Input: part model. Units: mm. Frame: model coordinates. A direction names the side the tool comes from. Give positions to 0.01 mm unless a question says otherwise; leave off trailing zeros. Write each loop counter-clockwise with the first axis right and the second up, starting at its lowest first coordinate (ties: lowest second). Pieces come first, ordered by that corner, then holes. Notation, with made-up numbers: (65, 50.5) -> (78, 50.5) arc R38 cw to (78, 89.5) -> close; hole circle Ø9 at (-1.75, 51.5). An arc over 180 degrees is marked (long way). Return JSON: item names as keys, results as strings. Group by question number.
Item 1: Section D-D, the plane y = -28.5. Return loops of the section in (x, z), then the cut area to 3 significant figures.
Item 2: Pin query (flat end, axial travel): P1, Ø4, axis at y = -44.5, z = 65.5, coming from the +X side; P2, Ø3, axis at y = -19.12, z = 75.53, coming from the +X side; P3, Ø2, axis at y = -19.12, z = 6, coming from the -X side. Return the tip coordinate at first contact, or that it passes through.
Item 3: Set-up query: faces 4 (the face through (1.85, -58.32, 1.63)), 5 (the face through (0.37, 0.61, -0.47)). Return all of +Z, -Z, +X, -X, +Y, -Y with unobstructed straight access to the full face (end or side cutting, diameter ignored); none if empty.
Item 4: Line query: line 1 (Z direction, x = 0.7, y = -19.12); line 2 (Y direction, x = -2, z = 6); line 3 (Z direction, x = -1.5, y = -19.12). Output: solid intervals per line, ascending. Write a range as [from, to].
Item 5: Mould query, pull axis Z, two halves, no side actions, for faces 1 (the face through (1.85, -58.22, 80)), 2 (the face through (-3, -29, 41)), 3 (the face through (0, -30, -3.25)). Classes: released by +Z, released by -Z, zero draft, split by the parting line, or undercut.
Item 6: Section A-A, the plane y = -19.12. Return loops of the section in (x, z).
Item 7: Section B-B, the plane x = -1. Return loops of the section in (y, z).
Item 8: Section C-C, the plane z = 54. Return loops of the section in (x, y), then the cut area to 3 significant figures.
from build123d import *

# Parameters (mm, degrees)
BOSS_EXTRUDE1_DEPTH = 3
SKETCH1_3_R         = 4.25
SKETCH1_3_R_2       = 1.25
BOSS_EXTRUDE2_DEPTH = 2
BOSS_EXTRUDE3_START = 3.64
BOSS_EXTRUDE3_DEPTH = 3.64
CUT_EXTRUDE1_REACH  = 107.747
SKETCH1_5_R         = 1.25


with BuildPart() as part:
    # Sketch1 → Boss-Extrude1 (new body)
    with BuildSketch(Plane(origin=(0, 0, 0), x_dir=(0, 0, -1), z_dir=(1, 0, 0))):
        with BuildLine():
            Line((-6, 3.25), (-75.53, 3.25))
            ThreePointArc((-75.53, 3.25), (-82.070737726, 0.540737726), (-84.78, -6))
            Line((-84.78, -6), (-84.78, -53.85))
            ThreePointArc((-84.78, -53.85), (-82.070737726, -60.390737726), (-75.53, -63.1))
            Line((-75.53, -63.1), (-6, -63.1))
            ThreePointArc((-6, -63.1), (0.540737726, -60.390737726), (3.25, -53.85))
            Line((3.25, -53.85), (3.25, -6))
            ThreePointArc((3.25, -6), (0.540737726, 0.540737726), (-6, 3.25))
        make_face()
    extrude(amount=-BOSS_EXTRUDE1_DEPTH)

    # Sketch1_3 → Boss-Extrude2 (add)
    # profile 1 of 4: a face of its own
    with BuildSketch(Plane(origin=(0, 0, 0), x_dir=(0, 0, -1), z_dir=(1, 0, 0))):
        with Locations(Location((-75.53, -19.12, 0), (0, 0, 180))):
            Circle(SKETCH1_3_R)
        with Locations((-75.53, -19.12)):
            Circle(SKETCH1_3_R_2, mode=Mode.SUBTRACT)
    # profile 2 of 4: a face of its own
    with BuildSketch(Plane(origin=(0, 0, 0), x_dir=(0, 0, -1), z_dir=(1, 0, 0))):
        with Locations(Location((-6, -19.12, 0), (0, 0, 180))):
            Circle(SKETCH1_3_R)
        with Locations((-6, -19.12)):
            Circle(SKETCH1_3_R_2, mode=Mode.SUBTRACT)
    # profile 3 of 4: a face of its own
    with BuildSketch(Plane(origin=(0, 0, 0), x_dir=(0, 0, -1), z_dir=(1, 0, 0))):
        with Locations(Location((-6, -42.05, 0), (0, 0, 180))):
            Circle(SKETCH1_3_R)
        with Locations((-6, -42.05)):
            Circle(SKETCH1_3_R_2, mode=Mode.SUBTRACT)
    # profile 4 of 4: a face of its own
    with BuildSketch(Plane(origin=(0, 0, 0), x_dir=(0, 0, -1), z_dir=(1, 0, 0))):
        with Locations(Location((-75.53, -42.05, 0), (0, 0, 180))):
            Circle(SKETCH1_3_R)
        with Locations((-75.53, -42.05)):
            Circle(SKETCH1_3_R_2, mode=Mode.SUBTRACT)
    extrude(amount=BOSS_EXTRUDE2_DEPTH)

    # Sketch1_4 → Boss-Extrude3 (add)
    with BuildSketch(Plane(origin=(0, 0, 0), x_dir=(0, 0, -1), z_dir=(1, 0, 0)).offset(BOSS_EXTRUDE3_START)):
        with BuildLine():
            ThreePointArc((-6, 3.25), (0.540737726, 0.540737726), (3.25, -6))
            Line((3.25, -6), (3.25, -53.85))
            ThreePointArc((3.25, -53.85), (0.540737726, -60.390737726), (-6, -63.1))
            Line((-6, -63.1), (-75.53, -63.1))
            ThreePointArc((-75.53, -63.1), (-82.070737726, -60.390737726), (-84.78, -53.85))
            Line((-84.78, -53.85), (-84.78, -6))
            ThreePointArc((-84.78, -6), (-82.070737726, 0.540737726), (-75.53, 3.25))
            Line((-75.53, 3.25), (-6, 3.25))
        make_face()
        with BuildLine():
            Line((-6, 0.25), (-75.53, 0.25))
            ThreePointArc((-75.53, 0.25), (-79.949417382, -1.580582618), (-81.78, -6))
            Line((-81.78, -6), (-81.78, -53.85))
            ThreePointArc((-81.78, -53.85), (-79.949417382, -58.269417382), (-75.53, -60.1))
            Line((-75.53, -60.1), (-6, -60.1))
            ThreePointArc((-6, -60.1), (-1.580582618, -58.269417382), (0.25, -53.85))
            Line((0.25, -53.85), (0.25, -6))
            ThreePointArc((0.25, -6), (-1.580582618, -1.580582618), (-6, 0.25))
        make_face(mode=Mode.SUBTRACT)
    extrude(amount=-BOSS_EXTRUDE3_DEPTH)

    # Sketch1_5 → Cut-Extrude1 (cut, up to next)
    with BuildSketch(Plane(origin=(0, 0, 0), x_dir=(0, 0, -1), z_dir=(1, 0, 0)), mode=Mode.PRIVATE) as cut_extrude1_sk1:
        with Locations(Location((-6, -19.12, 0), (0, 0, 180))):
            Circle(SKETCH1_5_R)
    cut_extrude1_tool1 = extrude(cut_extrude1_sk1.sketch, amount=-CUT_EXTRUDE1_REACH, mode=Mode.PRIVATE) & part.part
    # Sketch1_5 → Cut-Extrude1 (cut, up to next)
    with BuildSketch(Plane(origin=(0, 0, 0), x_dir=(0, 0, -1), z_dir=(1, 0, 0)), mode=Mode.PRIVATE) as cut_extrude1_sk2:
        with Locations(Location((-6, -42.05, 0), (0, 0, 180))):
            Circle(SKETCH1_5_R)
    cut_extrude1_tool2 = extrude(cut_extrude1_sk2.sketch, amount=-CUT_EXTRUDE1_REACH, mode=Mode.PRIVATE) & part.part
    # Sketch1_5 → Cut-Extrude1 (cut, up to next)
    with BuildSketch(Plane(origin=(0, 0, 0), x_dir=(0, 0, -1), z_dir=(1, 0, 0)), mode=Mode.PRIVATE) as cut_extrude1_sk3:
        with Locations(Location((-75.53, -19.12, 0), (0, 0, 180))):
            Circle(SKETCH1_5_R)
    cut_extrude1_tool3 = extrude(cut_extrude1_sk3.sketch, amount=-CUT_EXTRUDE1_REACH, mode=Mode.PRIVATE) & part.part
    # Sketch1_5 → Cut-Extrude1 (cut, up to next)
    with BuildSketch(Plane(origin=(0, 0, 0), x_dir=(0, 0, -1), z_dir=(1, 0, 0)), mode=Mode.PRIVATE) as cut_extrude1_sk4:
        with Locations(Location((-75.53, -42.05, 0), (0, 0, 180))):
            Circle(SKETCH1_5_R)
    cut_extrude1_tool4 = extrude(cut_extrude1_sk4.sketch, amount=-CUT_EXTRUDE1_REACH, mode=Mode.PRIVATE) & part.part
    add(cut_extrude1_tool1.solids().sort_by_distance((0, -19.12, 6))[0], mode=Mode.SUBTRACT)
    add(cut_extrude1_tool2.solids().sort_by_distance((0, -42.05, 6))[0], mode=Mode.SUBTRACT)
    add(cut_extrude1_tool3.solids().sort_by_distance((0, -19.12, 75.53))[0], mode=Mode.SUBTRACT)
    add(cut_extrude1_tool4.solids().sort_by_distance((0, -42.05, 75.53))[0], mode=Mode.SUBTRACT)


solid = part.part
Answer below:
{
 "1": {"outline": "(-3, -3.25) -> (3.64, -3.25) -> (3.64, -0.25) -> (0, -0.25) -> (0, 81.78) -> (3.64, 81.78) -> (3.64, 84.78) -> (-3, 84.78) -> close", "area": "286 mm2"},
 "2": {"P1": "stops at x = 0", "P2": "stops at x = 2", "P3": "passes through"},
 "3": {"face 4": "+X", "face 5": "-Z, +X, -X, +Y"},
 "4": {"line 1": "z = [-3.25, -0.25], [1.75, 4.75], [7.25, 10.25], [71.28, 74.28], [76.78, 79.78], [81.78, 84.78]", "line 2": "y = [-63.1, -43.3], [-40.8, -20.37], [-17.87, 3.25]", "line 3": "z = [-3.25, 4.75], [7.25, 74.28], [76.78, 84.78]"},
 "5": {"face 1": "undercut", "face 2": "zero draft", "face 3": "released by -Z"},
 "6": {"outline": "(-3, -3.25) -> (3.64, -3.25) -> (3.64, -0.25) -> (0, -0.25) -> (0, 1.75) -> (2, 1.75) -> (2, 4.75) -> (-3, 4.75) -> close; (-3, 7.25) -> (2, 7.25) -> (2, 10.25) -> (0, 10.25) -> (0, 71.28) -> (2, 71.28) -> (2, 74.28) -> (-3, 74.28) -> close; (-3, 76.78) -> (2, 76.78) -> (2, 79.78) -> (0, 79.78) -> (0, 81.78) -> (3.64, 81.78) -> (3.64, 84.78) -> (-3, 84.78) -> close"},
 "7": {"outline": "(-63.1, 6) arc R9.25 ccw to (-53.85, -3.25) -> (-6, -3.25) arc R9.25 ccw to (3.25, 6) -> (3.25, 75.53) arc R9.25 ccw to (-6, 84.78) -> (-53.85, 84.78) arc R9.25 ccw to (-63.1, 75.53) -> close; hole circle Ø2.5 at (-42.05, 6); hole circle Ø2.5 at (-42.05, 75.53); hole circle Ø2.5 at (-19.12, 6); hole circle Ø2.5 at (-19.12, 75.53)"},
 "8": {"outline": "(-3, -63.1) -> (3.64, -63.1) -> (3.64, -60.1) -> (0, -60.1) -> (0, 0.25) -> (3.64, 0.25) -> (3.64, 3.25) -> (-3, 3.25) -> close", "area": "221 mm2"}
}
